Autodesk Inventor part; units mm, degrees
ref_plane "Start plane" through (0, 0, 20) normal (0, 0, 1) x (1, 0, 0)
ref_plane "End plane" through (0, 0, 580) normal (0, 0, 1) x (1, 0, 0)
ref_plane "Work Plane4" through (-850, -13.6, 20) normal (0, 0, -1) x (-1, 0, 0)
ref_plane "Start plane" through (0, 0, 20) normal (0, 0, 1) x (1, 0, 0)
ref_plane "End plane" through (0, 0, 580) normal (0, 0, 1) x (1, 0, 0)
sketch "Sketch" plane through (0, 0, 0) normal (0, 0, 1) x (1, 0, 0)
  line L0 (-20, -13.6) -> (-20, 13.6)
  line L1 (-13.6, 20) -> (13.6, 20)
  line L2 (20, 13.6) -> (20, -13.6)
  line L3 (13.6, -20) -> (-13.6, -20)
  arc A0 (-20, -13.6) -> (-13.6, -20) centre (-13.6, -13.6) ccw
  arc A1 (-13.6, 20) -> (-20, 13.6) centre (-13.6, 13.6) ccw
  arc A2 (20, 13.6) -> (13.6, 20) centre (13.6, 13.6) ccw
  arc A3 (13.6, -20) -> (20, -13.6) centre (13.6, -13.6) ccw
  arc A4 (-13.6, 16.8) -> (-16.8, 13.6) centre (-13.6, 13.6) ccw
  line L4 (-13.6, 16.8) -> (13.6, 16.8)
  arc A5 (16.8, 13.6) -> (13.6, 16.8) centre (13.6, 13.6) ccw
  line L5 (16.8, 13.6) -> (16.8, -13.6)
  arc A6 (13.6, -16.8) -> (16.8, -13.6) centre (13.6, -13.6) ccw
  line L6 (13.6, -16.8) -> (-13.6, -16.8)
  arc A7 (-16.8, -13.6) -> (-13.6, -16.8) centre (-13.6, -13.6) ccw
  line L7 (-16.8, -13.6) -> (-16.8, 13.6)
  line L8 (0, 29.8557) -> (0, -29.8557) construction
  line L9 (-29.8557, 0) -> (29.8557, 0) construction
  dimension "d7" = 6.4
  dimension "d10" = 40
  dimension "d11" = 40
  dimension "d12" = 3.2
  dimension "d15" = 20
  dimension "d16" = 20
extrude "Body" add sketch "Sketch" along normal up to surface (560 mm away) from surface at 20
sketch "Sketch3" plane through (0, 0, 0) normal (0, 0, 1) x (1, 0, 0)
  line L0 (0, 0) -> (10, 0)
ref_plane "Work Plane3" through (0, 0, 0) normal (0, -1, 0) x (1, 0, 0)
sketch "Sketch4" plane through (0, 0, 0) normal (0, -1, 0) x (1, 0, 0)
  line L0 (-2, 20) -> (12, 20)
  line L1 (-2, 580) -> (12, 580)
  dimension "d18" = 560
ref_plane "Work Plane4" through (-850, -13.6, 20) normal (0, 0, -1) x (-1, 0, 0)
split "Split1" plane through (-850, -13.6, 20) removes the side toward (0, 0, -1)
ref_plane "Work Plane5" through (550, -13.6, 580) normal (0, 0, 1) x (1, 0, 0)
split "Split2" plane through (550, -13.6, 580) removes the side toward (0, 0, 1)
equation "\"d7\" = G_IR"
equation "\"d10\" = G_H"
equation "\"d11\" = G_W"
equation "\"d12\" = G_T"
equation "\"d15\" = 0.5 * d10"
equation "\"d16\" = 0.5 * d11"
equation "\"d3\" = G_L"
equation "\"G_W\" = 40"
equation "\"G_H\" = 40"
equation "\"G_T\" = 3.2"
equation "\"G_IR\" = 6.4"
equation "\"G_L\" = d18"
properties part number "BSI 40 x 40 x 3.2 00000004" material "Steel, Mild"
The listing builds one solid part. Answer for the finished solid, in the listing's coordinates (mm). A direction names the side the tool comes from. Give positions to 0.01 mm unless a question says otherwise; leave off trailing zeros. Loops run counter-clockwise (first coordinate to the right, second up) from the corner with the lowest first, then second, coordinate; pieces in that order, holes last. Notation, with made-up numbers: (-9.5, 31) - (-1.5, 31) arc R26 ccw to (-1.5, 58) - close; hole circle Ø2 at (87, 86). An arc over 180 degrees is marked (long way). Return JSON: item names as keys, results as strings. Group by question number.
1. Determine the mould class of faces 1 (the flat face through (-20, 0, 296)), 2 (the flat face through (0, -20, 296)), 3 (the flat face through (-16.8, 0, 296)) for opening direction X: pulls with the +X half, pulls with the -X half, needs draft (parallel to the pull), parting line crosses it, or undercut.
2. Which of the six approach directions +Z, -Z, +X, -X, +Y, -Y give full straight-line access (tool end or side, diameter ignored) to faces 4 (the flat face through (0, 20, 296)), 5 (the flat face through (16.8, 0, 296))?
3. Find section A-A (y = -4). Write down the section's boundary in (x, z).
4. Find section C-C (z = 59). Write down the section's boundary in (x, y), then the cut area to 3 significant figures.
5. Straight lines are drawn through the part: line 1 (Y direction, x = -13.5, z = 86.5); line 2 (X direction, y = 15.5, z = 389). For each, find the intervals that lie inside material, in ascending order. Write a range as [from, to].
Verdict:
{
 "1": {"face 1": "pulls with the -X half", "face 2": "needs draft", "face 3": "undercut"},
 "2": {"face 4": "+Z, -Z, +X, -X, +Y", "face 5": "+Z, -Z"},
 "3": {"outline": "(-20, 20) - (-16.8, 20) - (-16.8, 580) - (-20, 580) - close; (16.8, 20) - (20, 20) - (20, 580) - (16.8, 580) - close"},
 "4": {"outline": "(-20, -13.6) arc R6.4 ccw to (-13.6, -20) - (13.6, -20) arc R6.4 ccw to (20, -13.6) - (20, 13.6) arc R6.4 ccw to (13.6, 20) - (-13.6, 20) arc R6.4 ccw to (-20, 13.6) - close; hole (-16.8, -13.6) arc R3.2 ccw to (-13.6, -16.8) - (13.6, -16.8) arc R3.2 ccw to (16.8, -13.6) - (16.8, 13.6) arc R3.2 ccw to (13.6, 16.8) - (-13.6, 16.8) arc R3.2 ccw to (-16.8, 13.6) - close", "area": "445 mm^2"},
 "5": {"line 1": "y = [-20, -16.8], [16.8, 20]", "line 2": "x = [-19.71, -16.17], [16.17, 19.71]"}
}
